Verification items for the finished model (mm, model axes). Face numbers are marked on the shaded views. A direction names the side the tool comes from. Give positions to 0.01 mm unless a question says otherwise; leave off trailing zeros. Loops run counter-clockwise (first coordinate to the right, second up) from the corner with the lowest first, then second, coordinate; pieces in that order, holes last. Notation, with made-up numbers: (74.25, 61) - (126.25, 61) arc R3 cw to (126.25, 65) - close; hole circle Ø1 at (-16, 21). An arc over 180 degrees is marked (long way). One line per question, with ' | ' between items. Start each with the question number.
1. Depth check by flat-ended pin: pin 1 Ø4 at (x, y) = (52, 15) entering from +Z; pin 2 Ø2.5 at (x, y) = (36, 3) entering from +Z; pin 3 Ø1 at (x, z) = (43, 7.5) entering from +Y; pin 4 Ø10 at (y, z) = (59, 15) entering from -X. Enter the tip coordinate at first touch or a pass-through.
2. Section check D-D, the plane z = 12. Enter the section's corners in (x, y), then the cut area to 3 significant figures.
3. Thickness scan on line 1 along Z through (x, y) = (53, 70); line 2 along Y through (x, z) = (38.5, 2) (3 decimals); line 3 along Y through (x, z) = (37, 11). Record the ranges inside material, lowest first. Write a range as from..to.
4. Section check C-C, the plane y = 35.5. Enter the section's corners in (x, z), then the cut area to 3 significant figures.
5. Section check A-A, the plane z = -3. Enter the section's corners in (x, y) (3 decimals).
6. Tool access check on the marked faces 4, 5 and 6. Record the directions out of +Z, -Z, +X, -X, +Y, -Y that give a thin tool (end or side, any length) a straight path to the whole face; none if there is none.
7. Mould release check, pull along Z, two halves, no side actions. Record for the marked faces 1, 2 and 3: +Z half, -Z half, draft (parallel to the pull), parting line (faces both ways), or undercut.
Autodesk Fusion 360 part; units mm, degrees
sketch "Sketch1" plane through (0, 0, 0) normal (1, 0, 0) x (0, 1, 0)
  line L0 (0, 0) -> (8, 0)
  line L1 (8, 0) -> (24.8639, 36.1648)
  line L2 (0, 0) -> (0, 8)
  line L3 (0, 8) -> (-5, 8)
  line L4 (-5, 8) -> (-5, -7)
  line L5 (-5, -7) -> (11.814, -7)
  line L6 (11.814, -7) -> (31.9987, 36.2863)
  line L7 (32.1144, 40.7839) -> (32.8533, 40.7839)
  line L8 (39.4065, 37.3725) -> (65.575, 0)
  line L9 (37.0178, 40.7839) -> (86.8057, 40.7839) construction
  line L10 (65.575, 0) -> (73.575, 0)
  line L11 (73.575, 0) -> (73.575, 8)
  line L12 (73.575, 8) -> (78.575, 8)
  line L13 (78.575, 8) -> (78.575, -7)
  line L14 (78.575, -7) -> (62.3081, -7)
  line L15 (31.9987, 36.2863) -> (62.3081, -7)
  line L16 (35, 32) -> (86.0392, 32) construction
  arc A0 (32.1144, 40.7839) -> (24.8639, 36.1648) centre (32.1144, 32.7839) ccw
  arc A1 (39.4065, 37.3725) -> (32.8533, 40.7839) centre (32.8533, 32.7839) ccw
  point P0 (27.0178, 40.7839)
  dimension "d6" = 115
  dimension "d8" = 115
  dimension "d9" = 10
  dimension "d10" = 55
  dimension "d11" = 8
  dimension "d12" = 5
  dimension "d13" = 8
  dimension "d14" = 0
  dimension "d15" = 7
  dimension "d17" = 55
  dimension "d20" = 8
extrude "Extrude1" add sketch "Sketch1" along normal blind 60
fillet "Fillet1" radius 2.5 4 edges at (30, 0, 8) (30, -5, 8) (30, 73.575, 8) (30, 78.575, 8)
fillet "Fillet2" radius 10 1 edges at (30, 31.9987, 36.2863)
fillet "Fillet3" radius 5 2 edges at (30, 11.814, -7) (30, 62.3081, -7)
fillet "Fillet4" radius 2 2 edges at (30, -5, -7) (30, 78.575, -7)
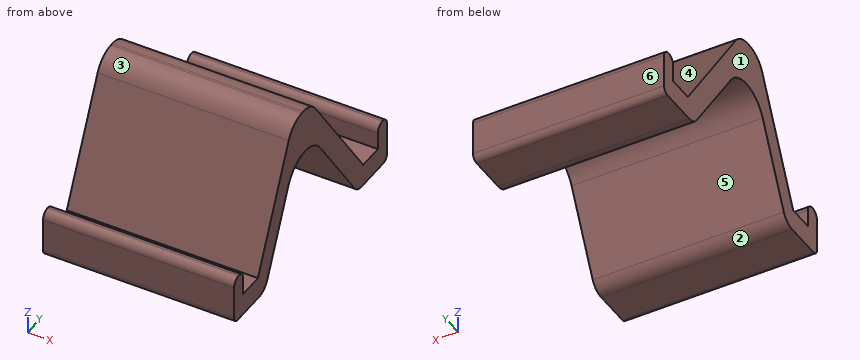
Results list:
1) pin 1: z = 19.3 | pin 2: z = 0 | pin 3: y = 78.08 | pin 4: x = 0
2) outline: (0, 13.6) - (60, 13.6) - (60, 20.67) - (0, 20.67) - close; (0, 49) - (60, 49) - (60, 57.17) - (0, 57.17) - close | area: 915 mm²
3) line 1: -7..0 | line 2: -5..0, 8.933..16.011, 56.006..64.175, 73.575..78.575 | line 3: 13.13..20.21, 49.7..57.87
4) outline: (0, 26.21) - (60, 26.21) - (60, 40.33) - (0, 40.33) - close | area: 848 mm²
5) outline: (0, -5) - (60, -5) - (60, 13.679) - (0, 13.679) - close; (0, 59.507) - (60, 59.507) - (60, 78.575) - (0, 78.575) - close
6) face 4: +Z, +X, -X | face 5: -Z, +X, -X | face 6: +Z, -Z, +X, -X, +Y
7) face 1: draft | face 2: -Z half | face 3: +Z half
